The model under review builds one solid part; all positions refer to its coordinate system, in mm. A direction names the side the tool comes from. Round coordinates to 2 decimals unless told otherwise and drop trailing zeros. Order: outer loops, then holes, each group sorted by start corner. A loop starts at its lowest first (then second) coordinate and runs counter-clockwise, first axis right, second up. Notation, with made-up numbers: M 13,17 L 20,17 A30 cw 20,44 Z; hole C 6,-16 d5. An arc over 180 degrees is marked long. Use a Markdown table: item, result. Add a question column.
1. The part is to be moulded in two halves that separate along Y. For faces 5 (the flat face through (12.688, -28, 15)), 6 (the flat face through (45.565, 27, 26)), 7 (the flat face through (38, -40.9, 12)), say which applies: +Y half, -Y half, draft (parallel to the pull), parting line (faces both ways), or undercut.
2. For faces 1 (the flat face through (-15.815, -6, 12)), 2 (the flat face through (84, 24, 22)), 3 (the flat face through (30.315, 24, 34)), 4 (the flat face through (6, -5, 15)), list the 3-axis set-ups (+Z, -Z, +X, -X, +Y, -Y) from which the entire face can be reached by the end or side of a thin tool; tool diameter is ignored.
3. Consider section D-D on z = 9. State the section outline as (x, y) points (3 decimals).
4. Consider section C-C on y = -12.5. State the section outline as (x, z) points (3 decimals).
5. Insertion check: P1, Ø3, axis at x = 6.5, y = -19, coming from the +Z side; P2, Ø1.6, axis at x = 12.5, z = 18.5, coming from the +Y side; P3, Ø3, axis at x = 34, y = 20.5, coming from the +Z side. Each pin has a flat end and moves straight along its axis. Give the tip position at first contact, or say it passes through.
6. Consider section B-B on x = 52. State the section outline as (y, z) points.
7. Consider section A-A on z = 29. State the section outline as (x, y) points (3 decimals).
8. To check wall thickness, follow probe 1 along X at (y, z) = (-17, 8) (3 decimals); probe 2 along Y at (x, z) = (32.45, 29); probe 3 along X at (y, z) = (19.5, 17) (3 decimals). State the ranges of each line that lie inside material, in increasing order.
from build123d import *

# Parameters (mm, degrees)
F0_W      = 110
F0_H      = 70
F0_W_2    = 13
F0_H_2    = 6
F0_W_3    = 53.87
F0_H_3    = 55
F0_W_4    = 2
F0_H_4    = 13
F1_DEPTH  = 25
F2_W      = 53.87
F2_H      = 55
F2_W_2    = 13
F2_H_2    = 6
F3_DEPTH  = 5
F4_W      = 2
F4_H      = 13
F5_DEPTH  = 15.5
F6_R      = 6.5
F6_R_2    = 4
F7_DEPTH  = 63.87
F8_W      = 10.25
F8_H      = 10.246950766
F8_H_2    = 5
F9_DEPTH  = 25
F11_DEPTH = 63.87
F12_W     = 63.8700000004
F12_H     = 64.876524617
F12_W_2   = 53.87
F12_H_2   = 55
F13_DEPTH = 1
F14_W     = 10.25
F14_H     = 10.246950766
F15_DEPTH = 3
F16_DEPTH = 3
F17_W     = 13
F17_H     = 6
F18_DEPTH = 5


# Not quite as in the source:
# - a feature names something its author has since deleted; it is built from what else it names


with BuildPart() as f1:
    # F0 (on Top) → F1 (new body)
    with BuildSketch(Plane.XY):
        with Locations((39.185, -5.9)):
            Rectangle(F0_W, F0_H)
        with Locations((6.18753814, -27.9975590407)):
            Rectangle(F0_W_2, F0_H_2, mode=Mode.SUBTRACT)
        with Locations((6.34376907, -17.9987795203)):
            Rectangle(F0_W_2, F0_H_2, mode=Mode.SUBTRACT)
        with Locations((6.5, -8)):
            Rectangle(F0_W_2, F0_H_2, mode=Mode.SUBTRACT)
        with Locations((62.25, -8.4)):
            Rectangle(F0_W_3, F0_H_3, mode=Mode.SUBTRACT)
        with Locations((6.5, 3)):
            Rectangle(F0_W_2, F0_H_2, mode=Mode.SUBTRACT)
        with Locations((1, 17.5)):
            Rectangle(F0_W_4, F0_H_4, mode=Mode.SUBTRACT)
        with Locations((6.5, 17.5)):
            Rectangle(F0_W_4, F0_H_4, mode=Mode.SUBTRACT)
        with Locations((12, 17.5)):
            Rectangle(F0_W_4, F0_H_4, mode=Mode.SUBTRACT)
    extrude(amount=F1_DEPTH)

    # F2 (on face) → F3 (join)
    with BuildSketch(Plane(origin=(0, 0, 0), x_dir=(1, 0, 0), z_dir=(0, 0, -1))):
        with Locations((62.25, 8.4)):
            Rectangle(F2_W, F2_H)
        with Locations((6.5, -3)):
            Rectangle(F2_W_2, F2_H_2)
        with Locations((6.5, 8)):
            Rectangle(F2_W_2, F2_H_2)
    extrude(amount=-F3_DEPTH)

    # F4 (on face) → F5 (join)
    with BuildSketch(Plane(origin=(0, 0, 0), x_dir=(1, 0, 0), z_dir=(0, 0, -1))):
        with Locations((12, -17.5)):
            Rectangle(F4_W, F4_H)
        with Locations((6.5, -17.5)):
            Rectangle(F4_W, F4_H)
        with Locations((1, -17.5)):
            Rectangle(F4_W, F4_H)
    extrude(amount=-F5_DEPTH)

    # F6 (on face) → F7 (join)
    with BuildSketch(Plane.YZ.offset(94.185)):
        with Locations((23.976524617, 29)):
            Circle(F6_R)
        with Locations((23.976524617, 29)):
            Circle(F6_R_2, mode=Mode.SUBTRACT)
    extrude(amount=-F7_DEPTH)

    # F8 (on face) → F9 (cut)
    with BuildSketch(Plane.XY.offset(25)):
        with Locations((40.44, 23.976524617)):
            Rectangle(F8_W, F8_H)
        with Locations((40.44, 16.353049234)):
            Rectangle(F8_W, F8_H_2)
        with Locations((40.44, 31.6)):
            Rectangle(F8_W, F8_H_2)
        with Locations((84.06, 16.353049234)):
            Rectangle(F8_W, F8_H_2)
        with Locations((84.06, 23.976524617)):
            Rectangle(F8_W, F8_H)
        with Locations((84.06, 31.6)):
            Rectangle(F8_W, F8_H_2)
    extrude(amount=F9_DEPTH, mode=Mode.SUBTRACT)

    # F10 (on face) → F11 (cut, through all)
    with BuildSketch(Plane.YZ.offset(94.185)):
        with BuildLine():
            ThreePointArc((23.976524617, 22.5), (21.1260860543, 23.1583392772), (18.853049234, 25))
            Line((18.853049234, 25), (-40.9, 25))
            Line((-40.9, 25), (-40.9, 22.5))
            Line((-40.9, 22.5), (23.976524617, 22.5))
        make_face()
    extrude(amount=-F11_DEPTH, mode=Mode.SUBTRACT)

    # F12 (on face) → F13 (join)
    with BuildSketch(Plane.XY.offset(22.5)):
        with Locations((62.2499999998, -8.4617376915)):
            Rectangle(F12_W, F12_H)
        with Locations((62.25, -8.4)):
            Rectangle(F12_W_2, F12_H_2, mode=Mode.SUBTRACT)
    extrude(amount=F13_DEPTH)

    # F14 (on face) → F15 (cut)
    with BuildSketch(Plane.XY.offset(25)):
        with Locations((40.44, 23.976524617)):
            Rectangle(F14_W, F14_H)
    extrude(amount=-F15_DEPTH, mode=Mode.SUBTRACT)

    # F16 (cut): a face of the model
    f16_faces = [f1.faces().sort_by_distance(p)[0] for p in [
        (84.06, 23.976524617, 25),
    ]]
    extrude(f16_faces, amount=-F16_DEPTH, mode=Mode.SUBTRACT)

    # F17 (on face) → F18 (join)
    with BuildSketch(Plane(origin=(0, 0, 0), x_dir=(1, 0, 0), z_dir=(0, 0, -1))):
        with Locations((6.34376907, 17.9987795203)):
            Rectangle(F17_W, F17_H)
        with Locations((6.18753814, 27.9975590407)):
            Rectangle(F17_W, F17_H)
    extrude(amount=-F18_DEPTH)


solid = f1.part
Answer block:
| question | item | result |
|---|---|---|
| 1 | face 5 | undercut |
| 1 | face 6 | draft |
| 1 | face 7 | -Y half |
| 2 | face 1 | +Z, -Z, -X, +Y, -Y |
| 2 | face 2 | +Z, +Y |
| 2 | face 3 | +Z, -X, +Y, -Y |
| 2 | face 4 | +Z |
| 3 | outline | M -15.815,-40.9 L 94.185,-40.9 L 94.185,29.1 L -15.815,29.1 Z; hole M -0.312,-30.998 L 12.688,-30.998 L 12.688,-24.998 L -0.312,-24.998 Z; hole M -0.156,-20.999 L 12.844,-20.999 L 12.844,-14.999 L -0.156,-14.999 Z; hole M 0,-11 L 13,-11 L 13,-5 L 0,-5 Z; hole M 0,0 L 13,0 L 13,6 L 0,6 Z; hole M 35.315,-35.9 L 89.185,-35.9 L 89.185,19.1 L 35.315,19.1 Z |
| 4 | outline | M -15.815,0 L 94.185,0 L 94.185,23.5 L 89.185,23.5 L 89.185,5 L 35.315,5 L 35.315,23.5 L 30.315,23.5 L 30.315,25 L -15.815,25 Z |
| 5 | P1 | z = 5 |
| 5 | P2 | y = 29.1 |
| 5 | P3 | z = 35.19 |
| 6 | outline | M -40.9,0 L 29.1,0 L 29.1,25 A6.5 ccw long 20.51,23.5 L 19.1,23.5 L 19.1,5 L -35.9,5 L -35.9,23.5 L -40.9,23.5 Z; hole C 23.98,29 d8 |
| 7 | outline | M 30.315,17.477 L 35.315,17.477 L 35.315,19.977 L 30.315,19.977 Z; M 30.315,27.977 L 35.315,27.977 L 35.315,30.477 L 30.315,30.477 Z; M 45.565,17.477 L 78.935,17.477 L 78.935,19.977 L 45.565,19.977 Z; M 45.565,27.977 L 78.935,27.977 L 78.935,30.477 L 45.565,30.477 Z; M 89.185,17.477 L 94.185,17.477 L 94.185,19.977 L 89.185,19.977 Z; M 89.185,27.977 L 94.185,27.977 L 94.185,30.477 L 89.185,30.477 Z |
| 8 | probe 1 | -15.815 to -0.156, 12.844 to 35.315, 89.185 to 94.185 |
| 8 | probe 2 | 17.48 to 19.98, 27.98 to 30.48 |
| 8 | probe 3 | -15.815 to 0, 2 to 5.5, 7.5 to 11, 13 to 94.185 |
